from build123d import *

# Parameters (mm, degrees)
F0_W     = 12
F0_H     = 10
F0_R     = 2
F1_DEPTH = 9
F2_DEPTH = 1
F4_DEPTH = 10
F6_DEPTH = 15
F7_R     = 2.5
F8_DEPTH = 1
F7_W     = 0.5
F7_H     = 2
F9_DEPTH = 2


with BuildPart() as f1:
    # F0 (on Right) → F1 (new body)
    with BuildSketch(Plane.YZ):
        Rectangle(F0_W, F0_H)
        Circle(F0_R, mode=Mode.SUBTRACT)
        Circle(F0_R)
    extrude(amount=F1_DEPTH)

    # F0 (on Right) → F2 (join)
    with BuildSketch(Plane.YZ):
        Circle(F0_R)
    extrude(amount=-F2_DEPTH)

    # F3 (on face) → F4 (join)
    with BuildSketch(Plane(origin=(-1, 0, 0), x_dir=(0, -1, 0), z_dir=(-1, 0, 0))):
        with BuildLine():
            ThreePointArc((-1, -1.118034), (0.612372, -1.369306), (1.5, 0))
            ThreePointArc((1.5, 0), (0.612372, 1.369306), (-1, 1.118034))
            Line((-1, 1.118034), (-1, -1.118034))
        make_face()
    extrude(amount=F4_DEPTH)

    # F5 (on face) → F6 (join)
    with BuildSketch(Plane.YZ.offset(9)):
        with BuildLine():
            Line((3.316625, 5), (-3.316625, 5))
            ThreePointArc((-3.316625, 5), (-5.286764, 2.837274), (-6, 0))
            ThreePointArc((-6, 0), (-5.286764, -2.837274), (-3.316625, -5))
            Line((-3.316625, -5), (3.316625, -5))
            ThreePointArc((3.316625, -5), (5.286764, -2.837274), (6, 0))
            ThreePointArc((6, 0), (5.286764, 2.837274), (3.316625, 5))
        make_face()
    extrude(amount=F6_DEPTH)

    # F7 (on face) → F8 (join)
    with BuildSketch(Plane.YZ.offset(24)):
        Circle(F7_R)
    extrude(amount=F8_DEPTH)

    # F7 (on face) → F9 (join)
    with BuildSketch(Plane.YZ.offset(24)):
        with Locations((-4, 0)):
            Rectangle(F7_W, F7_H)
        with Locations((4, 0)):
            Rectangle(F7_W, F7_H)
    extrude(amount=F9_DEPTH)


solid = f1.part
CAD build for the part. Positions are in the model's coordinates, mm. A direction names the side the tool comes from. Coordinates: 2 decimals unless noted, no trailing zeros. Write each loop counter-clockwise with the first axis right and the second up, starting at its lowest first coordinate (ties: lowest second). Pieces come first, ordered by that corner, then holes. Notation, with made-up numbers: M 37.5,11.5 L 60.5,11.5 A28 cw 60.5,49.5 Z; hole C 72.5,47.5 d5. An arc over 180 degrees is marked long. Answer as a JSON object with one key per item and string values. Group by question number.
1) Saw through at C-C (y = 5.25). Write the cut outline in (x, z).
2) Saw through at D-D (x = -5). Write the cut outline in (y, z), plus the area to 3 significant figures.
3) Pin check, flat tips, straight feed: pin 1 Ø1.6 at (x, z) = (25.5, 0.5) entering from +Y; pin 2 Ø1 at (x, z) = (25, -0.5) entering from -Y; pin 3 Ø5 at (y, z) = (0, -1) entering from +X. Stop position of each tip, or through.
4) Saw through at A-A (y = 0). Write the cut outline in (x, z), plus the area to 3 significant figures.
5) Wall check: line 1 (X direction, y = 5.75, z = -3.5); line 2 (X direction, y = 0.25, z = 3.5); line 3 (Y direction, x = 20, z = 4). Give the ranges that are in metal, low to high. Write a range as from..to.
6) Tool access for faces 1 (the face through (0, -0.1, 2.3)), 2 (the face through (9, -5, -4)), 3 (the face through (25, 4.25, 0)), 4 (the face through (25, -4.25, 0)), 5 (the face through (9, 5, -4)): list every direction of +Z, -Z, +X, -X, +Y, -Y with a clear straight run to the whole face (end or side of a thin tool).
7) Saw through at B-B (x = -0.5). Write the cut outline in (y, z), plus the area to 3 significant figures.
Values follow:
{
 "1": {"outline": "M 0,-5 L 9,-5 L 9,-2.9 L 24,-2.9 L 24,2.9 L 9,2.9 L 9,5 L 0,5 Z"},
 "2": {"outline": "M -1.5,0 A1.5 ccw 1,-1.12 L 1,1.12 A1.5 ccw Z", "area": "6.29 mm2"},
 "3": {"pin 1": "stops at y = 4.25", "pin 2": "stops at y = -4.25", "pin 3": "stops at x = 25"},
 "4": {"outline": "M -11,-1.5 L -1,-1.5 L -1,-2 L 0,-2 L 0,-5 L 24,-5 L 24,-2.5 L 25,-2.5 L 25,2.5 L 24,2.5 L 24,5 L 0,5 L 0,2 L -1,2 L -1,1.5 L -11,1.5 Z", "area": "279 mm2"},
 "5": {"line 1": "x = 0..9", "line 2": "x = 0..24", "line 3": "y = -4.47..4.47"},
 "6": {"face 1": "-X", "face 2": "-Z, +X, -Y", "face 3": "+Z, -Z, +X, +Y", "face 4": "+Z, -Z, +X, -Y", "face 5": "-Z, +X, +Y"},
 "7": {"outline": "C 0,0 d4", "area": "12.6 mm2"}
}
